```python
from build123d import *

# Parameters (mm, degrees)
EXTRUDE1_DEPTH    = 43.7642
HOLE1_D           = 19.05
HOLE1_DEPTH       = 0.254
HOLE2_D           = 20.574
HOLE2_DEPTH       = 4.826
SKETCH6_W         = 7.9375
SKETCH6_H         = 0.9906
SKETCH8_W         = 7.9375
SKETCH8_H         = 3.175
HOLE3_D           = 5.1816
HOLE3_DEPTH       = 10.922
CIRPATTERN1_COUNT = 2


with BuildPart() as part:
    # Sketch1 → Extrude1 (new body)
    with BuildSketch(Plane.XY.offset(43.7642)):
        with BuildLine():
            Line((20.070420221, 5.373106363), (12.3698, 34.1376))
            Line((12.3698, 34.1376), (-12.3698, 34.1376))
            Line((-12.3698, 34.1376), (-20.070420221, 5.373106363))
            ThreePointArc((-20.070420221, 5.373106363), (0, -20.7772), (20.070420221, 5.373106363))
        make_face()
    extrude(amount=-EXTRUDE1_DEPTH)

    # Hole1
    with Locations(Plane(origin=(0, 34.1376, 0), x_dir=(-1, 0, 0), z_dir=(0, 1, 0))):
        with Locations((0, 32.639)):
            Hole(HOLE1_D / 2, depth=HOLE1_DEPTH)

    # Hole2
    with Locations(Plane(origin=(0, 0, 0), x_dir=(-1, 0, 0), z_dir=(0, 0, -1))):
        with Locations((0, 0)):
            Hole(HOLE2_D / 2, depth=HOLE2_DEPTH)

    # Sketch7 → Revolve2 (revolve)
    with BuildSketch(Plane.XZ):
        Polygon((7.9375, 53.975), (0, 53.975), (0, 43.7642), (19.812, 43.7642), (19.812, 50.1142), (7.9375, 50.1142), align=None)
    revolve(axis=Axis((0, 0, 0), (0, 0, 1)))

    # Sketch6 → Revolve1 (revolve)
    with BuildSketch(Plane.XZ):
        with Locations((3.96875, 4.3307)):
            Rectangle(SKETCH6_W, SKETCH6_H)
    revolve(axis=Axis((0, 0, 0), (0, 0, 1)))

    # Sketch8 → Revolve3 (revolve)
    with BuildSketch(Plane(origin=(0, 0, 32.639), x_dir=(-1, 0, 0), z_dir=(0, 0, -1)), mode=Mode.PRIVATE) as revolve3_sk:
        with Locations((-3.96875, 35.4711)):
            Rectangle(SKETCH8_W, SKETCH8_H)
    revolve(revolve3_sk.sketch.rotate(Axis((0, 0, 32.639), (0, 1, 0)), 270), axis=Axis((0, 0, 32.639), (0, 1, 0)))  # turned: the seam where the file's is

    # Sketch9 → Cut-Revolve1 (revolve, cut)
    with BuildSketch(Plane(origin=(0, 0, 11.9888), x_dir=(-1, 0, 0), z_dir=(0, 0, -1)), mode=Mode.PRIVATE) as cut_revolve1_sk:
        Polygon((-4.9784, 13.3096), (0, 13.3096), (0, 34.1376), (-9.525, 34.1376), (-9.525, 33.8836), (-6.1849, 33.8836), (-5.642306865, 31.3309), (-4.9784, 30.666993135), align=None)
    revolve(cut_revolve1_sk.sketch.rotate(Axis((0, 13.3096, 11.9888), (0, 1, 0)), 270), axis=Axis((0, 13.3096, 11.9888), (0, 1, 0)), mode=Mode.SUBTRACT)  # turned: the seam where the file's is

    # Sketch10 → Cut-Revolve2 (revolve, cut)
    with BuildSketch(Plane.XY.offset(32.639), mode=Mode.PRIVATE) as cut_revolve2_sk:
        Polygon((6.1849, 33.8836), (0, 33.8836), (0, 20.4216), (4.9784, 20.4216), (4.9784, 30.666993135), (5.642306865, 31.3309), align=None)
    revolve(cut_revolve2_sk.sketch.rotate(Axis((0, 33.8836, 32.639), (0, -1, 0)), 270), axis=Axis((0, 33.8836, 32.639), (0, -1, 0)), mode=Mode.SUBTRACT)  # turned: the seam where the file's is

    # Hole3
    with Locations(Plane(origin=(0, 0, 0), x_dir=(-1, 0, 0), z_dir=(0, 0, -1))):
        with Locations((-15.875, 0)):
            hole3 = Hole(HOLE3_D / 2, depth=HOLE3_DEPTH)

    # CirPattern1: Hole3 ×2 about axis
    cirpattern1_axis = Axis((0, 0, 0), (0, 0, 1))
    for i in range(1, CIRPATTERN1_COUNT):
        add(hole3.rotate(cirpattern1_axis, i * 360 / CIRPATTERN1_COUNT), mode=Mode.SUBTRACT)

    # Sketch15 → Hole5 (revolve, cut)
    with BuildSketch(Plane(origin=(0, 0, 3.8354), x_dir=(0, 1, 0), z_dir=(1, 0, 0))):
        Polygon((0, 0), (0, 50.1396), (3.9751, 50.1396), (3.9751, 35.761676477), (5.1562, 35.052), (5.1562, 0), align=None)
    revolve(axis=Axis((0, 0, -2.294623899), (0, 0, 1)), mode=Mode.SUBTRACT)


solid = part.part
```
Geometry: final body of the model. Coordinates: model frame, mm. A direction names the side the tool comes from. Coordinates: 2 decimals unless noted, no trailing zeros. Order: outer loops, then holes, each group sorted by start corner. A loop starts at its lowest first (then second) coordinate and runs counter-clockwise, first axis right, second up. Notation, with made-up numbers: (-12.75, 58.5) -> (8.25, 58.5) arc R15 cw to (8.25, 83.5) -> close; hole circle Ø4 at (53, -27.75). An arc over 180 degrees is marked (long way). Use CSV: the item, a comma, the result in double quotes.
1) Section A-A on x = 0. State how many separate pieces and enclosed holes the cut face has, then the cut area to 3 significant figures.
Findings:
separate pieces,"2"
enclosed holes,"1"
area,"1,840 mm^2"
2) Mould query, pull axis Z, two halves, no side actions, for faces 5 (the flat face through (-16.166, 19.957, 22.188)), 6 (the flat face through (-4, 33.884, 40)), 7 (the flat face through (0, -9, 50.114)). Classes: +Z half, -Z half, draft (parallel to the pull), parting line (faces both ways), or undercut.
Findings:
face 5,"draft"
face 6,"undercut"
face 7,"+Z half"
3) Section B-B on z = 43. Output: boundary loops of the cut face in (x, y).
Findings:
outline,"(-20.07, 5.37) arc R20.78 ccw (long way) to (20.07, 5.37) -> (12.37, 34.14) -> (-12.37, 34.14) -> close; hole circle Ø7.95 at (0, 0)"
4) Access query for faces 1 (the cylindrical face through (-0.53, -20.77, 22.19)), 2 (the flat face through (0, 33.884, 33)), 3 (the flat face through (-6.2, 33.884, 14)), 4 (the flat face through (-16, 0, 10.922)). Directions: +Z, -Z, +X, -X, +Y, -Y. A direction counts if a zero-diameter tool reaches every point of the face in a straight line with its end or side. Return the directions, or none.
Findings:
face 1,"+Z, -Z"
face 2,"none"
face 3,"+Y"
face 4,"-Z"
5) Section C-C on y = 19. Output: boundary loops of the cut face in (x, z), then the cut area to 3 significant figures.
Findings:
outline,"(-16.42, 0) -> (16.42, 0) -> (16.42, 43.76) -> (5.61, 43.76) -> (5.61, 50.11) -> (-5.61, 50.11) -> (-5.61, 43.76) -> (-16.42, 43.76) -> close; hole circle Ø9.96 at (0, 11.99)"
area,"1,430 mm^2"
6) Pin query (flat end, axial travel): pin 1 Ø4 at (x, y) = (16.5, 0.5) entering from -Z; pin 2 Ø1 at (x, z) = (-10.5, 6) entering from +Y; pin 3 Ø16.5 at (x, y) = (0, 0) entering from -Z; pin 4 Ø12 at (y, z) = (22.5, 30) entering from +X. Return the tip coordinate at first contact, or that it passes through.
Findings:
pin 1,"stops at z = 0"
pin 2,"stops at y = 34.14"
pin 3,"stops at z = 3.84"
pin 4,"stops at x = 17.09"
7) Line query: line 1 (Z direction, x = 2.5, y = 21.5); line 2 (Y direction, x = -4, z = 4.5); line 3 (Y direction, x = 6, z = 4). Output: solid intervals per line, ascending.
Findings:
line 1,"z = 0 to 7.68, 16.29 to 28.33, 36.94 to 43.76"
line 2,"y = -20.39 to -9.48, -6.86 to -3.25, 3.25 to 6.86, 9.48 to 33.88"
line 3,"y = -19.89 to -8.36, -5.2 to 5.2, 8.36 to 34.14"
8) Section D-D on x = -14.5. Output: boundary loops of the cut face in (y, z), then the cut area to 3 significant figures.
Findings:
outline,"(-14.88, 0) -> (-2.2, 0) -> (-2.2, 10.92) -> (2.2, 10.92) -> (2.2, 0) -> (26.18, 0) -> (26.18, 43.76) -> (13.5, 43.76) -> (13.5, 50.11) -> (-13.5, 50.11) -> (-13.5, 43.76) -> (-14.88, 43.76) -> close"
area,"1,920 mm^2"
